from build123d import *

# Parameters (mm, degrees)
SKETCH1_W            = 20
SKETCH1_H            = 6.35
SKETCH1_W_2          = 6.35
SKETCH1_H_2          = 20
BOSS_EXTRUDE1_DEPTH  = 38.1
SKETCH2_W            = 42.3
SKETCH2_H            = 10.16
SKETCH2_W_2          = 15.95
SKETCH2_H_2          = 26.35
SKETCH2_W_3          = 10.16
SKETCH2_H_3          = 52.46
BOSS_EXTRUDE3_DEPTH  = 6.35
SKETCH3_R            = 1.7
SKETCH3_R_2          = 15.431993428
CUT_EXTRUDE1_DEPTH   = 6.35
BOSS_EXTRUDE5_DEPTH  = 2.54
SKETCH6_W            = 10.16
SKETCH6_H            = 26.35
BOSS_EXTRUDE6_DEPTH  = 6.35
BOSS_EXTRUDE7_DEPTH  = 2.54
BOSS_EXTRUDE8_DEPTH  = 2.54
M4_CLEARANCE_HOLE2_D = 4.5
M4_CLEARANCE_HOLE3_D = 4.5


with BuildPart() as part:
    # Sketch1 → Boss-Extrude1 (new body)
    with BuildSketch(Plane(origin=(0, 0, 0), x_dir=(1, 0, 0), z_dir=(0, 1, 0))):
        with Locations((10, -3.175)):
            Rectangle(SKETCH1_W, SKETCH1_H)
        with Locations((-3.175, -3.175)):
            Rectangle(SKETCH1_W_2, SKETCH1_H)
        with Locations((-3.175, 10)):
            Rectangle(SKETCH1_W_2, SKETCH1_H_2)
    extrude(amount=BOSS_EXTRUDE1_DEPTH)

    # Sketch2 → Boss-Extrude3 (add)
    with BuildSketch(Plane.XZ):
        Polygon((-6.35, 6.35), (20, 6.35), (20, 48.65), (-22.3, 48.65), (-22.3, 6.35), align=None)
        with Locations((-1.15, 53.73)):
            Rectangle(SKETCH2_W, SKETCH2_H)
        with Locations((-14.325, -6.825)):
            Rectangle(SKETCH2_W_2, SKETCH2_H_2)
        with Locations((-27.38, 32.58)):
            Rectangle(SKETCH2_W_3, SKETCH2_H_3)
    extrude(amount=-BOSS_EXTRUDE3_DEPTH)

    # Sketch3 → Cut-Extrude1 (cut)
    with BuildSketch(Plane(origin=(0, 6.35, 0), x_dir=(1, 0, 0), z_dir=(0, 1, 0))):
        with Locations(Location((4.19, -22.16, 0), (0, 0, 270))):
            Circle(SKETCH3_R)
        with Locations(Location((-26.81, -53.16, 0), (0, 0, 270))):
            Circle(SKETCH3_R)
        with Locations(Location((-26.81, -22.16, 0), (0, 0, 270))):
            Circle(SKETCH3_R)
        with Locations(Location((-11.314321333, -37.591993428, 0), (0, 0, 270))):
            Circle(SKETCH3_R_2)
        with Locations(Location((4.19, -53.16, 0), (0, 0, 270))):
            Circle(SKETCH3_R)
    extrude(amount=-CUT_EXTRUDE1_DEPTH, mode=Mode.SUBTRACT)

    # Sketch5 → Boss-Extrude5 (add)
    with BuildSketch(Plane(origin=(20, 0, 0), x_dir=(0, 0, -1), z_dir=(1, 0, 0))):
        Polygon((-6.35, 38.1), (-58.81, 6.35), (-6.35, 6.35), align=None)
    extrude(amount=-BOSS_EXTRUDE5_DEPTH)

    # Sketch6 → Boss-Extrude6 (add)
    with BuildSketch(Plane(origin=(0, 6.35, 0), x_dir=(1, 0, 0), z_dir=(0, 1, 0))):
        with Locations((-27.38, 6.825)):
            Rectangle(SKETCH6_W, SKETCH6_H)
    extrude(amount=-BOSS_EXTRUDE6_DEPTH)

    # Sketch7 → Boss-Extrude7 (add)
    with BuildSketch(Plane(origin=(0, 0, -20), x_dir=(-1, 0, 0), z_dir=(0, 0, -1))):
        Polygon((6.35, 38.1), (32.46, 6.35), (6.35, 6.35), align=None)
    extrude(amount=-BOSS_EXTRUDE7_DEPTH)

    # Sketch8 → Boss-Extrude8 (add)
    with BuildSketch(Plane.XY.offset(6.35)):
        Polygon((-6.35, 38.1), (-32.46, 6.35), (-6.35, 6.35), align=None)
    extrude(amount=-BOSS_EXTRUDE8_DEPTH)

    # M4 Clearance Hole2 (through all)
    with Locations(Plane.ZY.offset(6.35)):
        with Locations((-10, 30.1625), (-10, 14.2875)):
            Hole(M4_CLEARANCE_HOLE2_D / 2)

    # M4 Clearance Hole3 (through all)
    with Locations(Plane.XY.offset(6.35)):
        with Locations((10, 30.1625), (10, 14.2875)):
            Hole(M4_CLEARANCE_HOLE3_D / 2)


solid = part.part
Here's how the part is built. I have some questions about the finished solid (model axes, mm). A direction names the side the tool comes from. Coordinates: 2 decimals unless noted, no trailing zeros. Order: outer loops, then holes, each group sorted by start corner. A loop starts at its lowest first (then second) coordinate and runs counter-clockwise, first axis right, second up. Notation, with made-up numbers: M -10.5,15.25 L 13.5,15.25 A31 ccw 13.5,51.25 Z; hole C 74,-30.5 d4. An arc over 180 degrees is marked long. Answer as CSV lines item,"result". Start each with the question number.
1. I want a section at D-D, the plane y = 15.5. Write out the boundary of the cut face in (x, z), and give its area (3 significant figures).
2. We'd pull the mould along Z, two halves only. Please class faces 1 (the flat face through (10, 19, 0)), 2 (the flat face through (-20, 6.35, -7)), 3 (the flat face through (-7, 0, 19)), 4 (the flat face through (18.75, 22.45, 32.21)): released by +Z, released by -Z, zero draft, split by the parting line, or undercut.
3. I want a section at C-C, the plane z = 32.5. Write out the boundary of the cut face in (x, y).
4. I need wall thicknesses on line 1 (Y direction, x = -4.25, z = -10); line 2 (Z direction, x = -7, y = 27.5). Which ranges of each line are inside material? Lowest first, please. Write a range as [from, to].
5. For pin 1 (3 mm diameter, centred on x = -26.81, z = 22.16, fed in from +Y); pin 2 (2 mm diameter, centred on y = 17, z = 2, fed in from -X); pin 3 (1 mm diameter, centred on x = -3, z = 18, fed in from +Y); pin 4 (9.5 mm diameter, centred on y = 25, z = 22, fed in from -X), each with a flat end and sliding along its axis, tell me the tip position at first contact or that it passes through.
6. I want a section at B-B, the plane x = 10. Write out the boundary of the cut face in (y, z).
7. I want a section at A-A, the plane z = -10. Write out the boundary of the cut face in (x, y).
8. On a 3-axis mill with a long thin cutter (end or side, diameter ignored), from which of +Z, -Z, +X, -X, +Y, -Y can I reach the whole of each face in a straight line? I mean faces 5 (the flat face through (17.46, 15, 21)), 6 (the flat face through (-2, 38.1, -1)), 7 (the flat face through (-14, 15, -17.46)), 8 (the flat face through (0, 19, -10)). Say none if no direction works.
Recorded:
1,outline,"M -24.94,-20 L 0,-20 L 0,-11.9 L -6.35,-11.9 L -6.35,-17.46 L -24.94,-17.46 Z; M -24.94,3.81 L -6.35,3.81 L -6.35,-8.1 L 0,-8.1 L 0,0 L 8.1,0 L 8.1,6.35 L -24.94,6.35 Z; M 11.9,0 L 20,0 L 20,43.69 L 17.46,43.69 L 17.46,6.35 L 11.9,6.35 Z"
1,area,"435 mm2"
2,face 1,"released by -Z"
2,face 2,"undercut"
2,face 3,"zero draft"
2,face 4,"released by +Z"
3,outline,"M -32.46,0 L -25.88,0 L -25.88,6.35 L -32.46,6.35 Z; M 3.25,0 L 20,0 L 20,22.27 L 17.46,22.27 L 17.46,6.35 L 3.25,6.35 Z"
4,line 1,"y = [0, 12.04], [16.54, 27.91], [32.41, 38.1]"
4,line 2,"z = [-20, -17.46], [3.81, 6.35]"
5,pin 1,"passes through"
5,pin 2,"stops at x = -6.35"
5,pin 3,"stops at y = 6.35"
5,pin 4,"stops at x = 17.46"
6,outline,"M 0,0 L 12.04,0 L 12.04,6.35 L 6.35,6.35 L 6.35,58.81 L 0,58.81 Z; M 16.54,0 L 27.91,0 L 27.91,6.35 L 16.54,6.35 Z; M 32.41,0 L 38.1,0 L 38.1,6.35 L 32.41,6.35 Z"
7,outline,"M -32.46,0 L 0,0 L 0,12.04 L -6.35,12.04 L -6.35,6.35 L -32.46,6.35 Z; M -6.35,16.54 L 0,16.54 L 0,27.91 L -6.35,27.91 Z; M -6.35,32.41 L 0,32.41 L 0,38.1 L -6.35,38.1 Z"
8,face 5,"+Z, -X, +Y"
8,face 6,"+Z, -Z, +X, -X, +Y"
8,face 7,"-X, +Y"
8,face 8,"-Z, +X, +Y, -Y"
